Verification items for the finished model (mm, model axes). Round coordinates to 2 decimals unless told otherwise and drop trailing zeros. Order: outer loops, then holes, each group sorted by start corner. A loop starts at its lowest first (then second) coordinate and runs counter-clockwise, first axis right, second up. Notation, with made-up numbers: M 51,20 L 99,20 A25 cw 99,55 Z; hole C 52.5,81 d11. An arc over 180 degrees is marked long. Use one line per item in the form item = value. Start each with the question number.
Item 1: Cross-section at D-D on z = 1.5. Enter the section's corners in (x, y), then the cut area to 3 significant figures.
Item 2: Go/stop test with flat-tipped pins: pin 1 Ø1.5 at (x, z) = (-12, 7) entering from +Y; pin 2 Ø1 at (x, z) = (-6, 7.5) entering from -Y; pin 3 Ø2 at (x, z) = (8, 9.5) entering from +Y. Record where each tip stops, or that it passes through.
Item 3: Cross-section at A-A on y = 0. Enter the section's corners in (x, z).
Item 4: Thickness scan on probe 1 along Y at (x, z) = (0, -0.7); probe 2 along Z at (x, y) = (1.5, -1); probe 3 along Y at (x, z) = (0, 7.25). Record the ranges inside material, lowest first. Write a range as [from, to].
Item 5: Cross-section at C-C on z = 7. Enter the section's corners in (x, y).
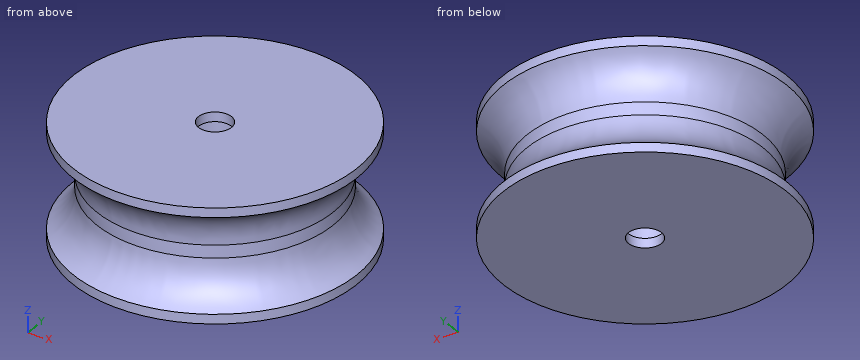
from build123d import *

# Parameters (mm, degrees)
SKETCH1_R                  = 12.5
BOSS_EXTRUDE1_DEPTH        = 10
F_6_0_204_DIAMETER_SLOT2_D = 5.1816
SKETCH10_R                 = 15
BOSS_EXTRUDE2_DEPTH        = 1
BOSS_EXTRUDE3_START        = 1
SKETCH12_R                 = 15
BOSS_EXTRUDE3_DEPTH        = 1
SKETCH13_R                 = 1.75
CUT_EXTRUDE1_DEPTH         = 25.372115214
FILLET4_R                  = 5
FILLET5_R                  = 5


with BuildPart() as part:
    # Sketch1 → Boss-Extrude1 (new body)
    with BuildSketch(Plane.XY):
        Circle(SKETCH1_R)
    extrude(amount=BOSS_EXTRUDE1_DEPTH)

    # #6 (0.204) Diameter Slot2 (through all)
    with Locations(Plane.XY.offset(10)):
        with Locations((0, 0)):
            Hole(F_6_0_204_DIAMETER_SLOT2_D / 2)

    # Sketch10 → Boss-Extrude2 (add)
    with BuildSketch(Plane(origin=(0, 0, 0), x_dir=(-1, 0, 0), z_dir=(0, 0, -1))):
        Circle(SKETCH10_R)
    extrude(amount=BOSS_EXTRUDE2_DEPTH)

    # Sketch12 → Boss-Extrude3 (add)
    with BuildSketch(Plane.XY.offset(10).offset(BOSS_EXTRUDE3_START)):
        with Locations(Location((0, 0, 0), (0, 0, 180))):
            Circle(SKETCH12_R)
    extrude(amount=-BOSS_EXTRUDE3_DEPTH)

    # Sketch13 → Cut-Extrude1 (cut, through all)
    with BuildSketch(Plane.XY.offset(11)):
        Circle(SKETCH13_R)
    extrude(amount=-CUT_EXTRUDE1_DEPTH, mode=Mode.SUBTRACT)

    # Fillet4
    # the kernel refuses this fillet: 5 mm, written as the material it adds along each edge
    with BuildSketch(Plane(origin=(0, 0, 10), x_dir=(1, 0, 0), z_dir=(0, -1, 0))) as fillet4_piece_1:
        with BuildLine():
            CenterArc((17.5, -4.330127019), FILLET4_R, 120, 60)
            Line((12.5, -4.330127019), (12.4, -4.330127019))
            Line((12.4, -4.330127019), (12.4, 0))
            Line((12.4, 0), (12.5, 0.1))
            ThreePointArc((12.5, 0.1), (13.75, 0.1), (14.95, 0.08660254))
            Line((14.95, 0.08660254), (15, 0))
        make_face()
    revolve(axis=Axis((0, 0, 10), (0, 0, 1)))

    # Fillet5
    # the kernel refuses this fillet: 5 mm, written as the material it adds along each edge
    with BuildSketch(Plane(origin=(0, 0, 0), x_dir=(1, 0, 0), z_dir=(0, -1, 0))) as fillet5_piece_1:
        with BuildLine():
            CenterArc((17.5, 4.330127019), FILLET5_R, 180, 60)
            Line((15, 0), (14.95, -0.08660254))
            ThreePointArc((14.95, -0.08660254), (13.75, -0.1), (12.5, -0.1))
            Line((12.5, -0.1), (12.4, 0))
            Line((12.4, 0), (12.4, 4.330127019))
            Line((12.4, 4.330127019), (12.5, 4.330127019))
        make_face()
    revolve(axis=Axis((0, 0, 0), (0, 0, 1)))


solid = part.part
Output values:
q1.outline = C 0,0 d26.76; hole C 0,0 d5.18
q1.area = 541 mm2
q2.pin_1 = 5.93
q2.pin_2 = -11.71
q2.pin_3 = 13.19
q3.outline = M -15,-1 L -1.75,-1 L -1.75,0 L -2.59,0 L -2.59,10 L -1.75,10 L -1.75,11 L -15,11 L -15,10 A5 cw -12.5,5.67 L -12.5,4.33 A5 cw -15,0 Z; M 1.75,-1 L 15,-1 L 15,0 A5 cw 12.5,4.33 L 12.5,5.67 A5 cw 15,10 L 15,11 L 1.75,11 L 1.75,10 L 2.59,10 L 2.59,0 L 1.75,0 Z
q4.probe_1 = [-15, -1.75], [1.75, 15]
q4.probe_2 = [-1, 0], [10, 11]
q4.probe_3 = [-12.76, -2.59], [2.59, 12.76]
q5.outline = C 0,0 d25.36; hole C 0,0 d5.18
